The model under review builds one solid part; all positions refer to its coordinate system, in mm. A direction names the side the tool comes from. Round coordinates to 2 decimals unless told otherwise and drop trailing zeros. Write each loop counter-clockwise with the first axis right and the second up, starting at its lowest first coordinate (ties: lowest second). Pieces come first, ordered by that corner, then holes.
Item 1: Add section B-B (x = 0.5). Give the boundary of the cut face in (y, z).
Item 2: Machinability: for faces 1 (the face through (-2, 5, 2)), 2 (the face through (2.024, 3.028, 1.29)), which of the approach directions +Z, -Z, +X, -X, +Y, -Y give a long, thin tool a straight path to every point of the face, cutting with its end or side? Answer none if there is none.
Item 3: Add section A-A (z = 0). Give the boundary of the cut face in (x, y), plus the area to 3 significant figures.
Item 4: Add section C-C (y = 2.05). Give the boundary of the cut face in (x, z).
Item 5: Draft analysis for pull direction X (two halves, no side actions). For faces 3 (the face through (-2, 1, 0)), 4 (the face through (-3.905, 2.465, -0.867)), 5 (the face through (0, 0, 2)), state which applies: +X half, -X half, draft (parallel to the pull), parting line (faces both ways), or undercut.
Item 6: To check wall thickness, follow L1, parallel to X at y = 3.6, z = 0; L2, parallel to X at y = 0.3, z = 0; L3, parallel to Z at x = -0.75, y = 4.45. State the ranges of each line that lie inside material, in increasing order.
Item 7: Add section D-D (z = -2). Give the boundary of the cut face in (x, y), plus the area to 3 significant figures.
Item 8: Clearance check with a flat-ended pin moving along its axis: pin 1 Ø2 at (y, z) = (3, -3) entering from +X. State where the tip first meets the part, or that it passes through.
```python
from build123d import *

# Parameters (mm, degrees)
ESQUISSE1_R             = 4
BOSS_EXTRU_1_DEPTH      = 5
ESQUISSE3_R             = 1.5
ENL_V_MAT_EXTRU_2_DEPTH = 8.549834435
ESQUISSE2_R             = 2.4
ENL_V_MAT_EXTRU_3_DEPTH = 4


with BuildPart() as part:
    # Esquisse1 → Boss.-Extru.1 (new body)
    with BuildSketch(Plane(origin=(0, 0, 0), x_dir=(1, 0, 0), z_dir=(0, 1, 0))):
        with Locations(Location((0, 0, 0), (0, 0, 270))):
            Circle(ESQUISSE1_R)
    extrude(amount=BOSS_EXTRU_1_DEPTH)

    # Esquisse3 → Enlèv. mat.-Extru.2 (cut, through all)
    with BuildSketch(Plane.XZ):
        with Locations(Location((0, 0, 0), (0, 0, 270))):
            Circle(ESQUISSE3_R)
    extrude(amount=-ENL_V_MAT_EXTRU_2_DEPTH, mode=Mode.SUBTRACT)

    # Esquisse2 → Enlèv. mat.-Extru.3 (cut)
    with BuildSketch(Plane(origin=(0, 5, 0), x_dir=(1, 0, 0), z_dir=(0, 1, 0))):
        with Locations(Location((0, 0, 0), (0, 0, 270))):
            Circle(ESQUISSE2_R)
    extrude(amount=-ENL_V_MAT_EXTRU_3_DEPTH, mode=Mode.SUBTRACT)


solid = part.part
```
Numbers:
1. outline: (0, -3.97) - (5, -3.97) - (5, -2.35) - (1, -2.35) - (1, -1.41) - (0, -1.41) - close; (0, 1.41) - (1, 1.41) - (1, 2.35) - (5, 2.35) - (5, 3.97) - (0, 3.97) - close
2. face 1: +Z, -Z, +X, -X, +Y
2. face 2: +Y
3. outline: (-4, 0) - (-1.5, 0) - (-1.5, 1) - (-2.4, 1) - (-2.4, 5) - (-4, 5) - close; (1.5, 0) - (4, 0) - (4, 5) - (2.4, 5) - (2.4, 1) - (1.5, 1) - close
3. area: 17.8 mm2
4. outline: circle Ø8 at (0, 0); hole circle Ø4.8 at (0, 0)
5. face 3: undercut
5. face 4: parting line
5. face 5: draft
6. L1: x = -4 to -2.4, 2.4 to 4
6. L2: x = -4 to -1.5, 1.5 to 4
6. L3: z = -3.93 to -2.28, 2.28 to 3.93
7. outline: (-3.46, 0) - (3.46, 0) - (3.46, 5) - (1.33, 5) - (1.33, 1) - (-1.33, 1) - (-1.33, 5) - (-3.46, 5) - close
7. area: 24.0 mm2
8. pin 1: stops at x = 3.46
